from build123d import *

# Parameters (mm, degrees)
F1_DEPTH  = 3
F3_DEPTH  = 2
F4_R      = 1.5
F5_DEPTH  = 3
F6_SIZE   = 1
F7_R      = 1
F9_DEPTH  = 1.0010001
F10_R     = 1.49999
F11_W     = 6
F11_H     = 1.5
F12_DEPTH = 2.5


# Not quite as in the source:
# - a fillet or chamfer is up to 0.001 mm smaller than in the source, because OpenCascade refuses the exact size


with BuildPart() as f1:
    # F0 (on Top) → F1 (new body)
    with BuildSketch(Plane.XY):
        Polygon((4, 20), (-4, 20), (-4, 14.4568322948), (-17.7288018167, 0), (0, -18.8113879412), (17.1686839312, 0), (4, 14.4568322948), align=None)
    extrude(amount=F1_DEPTH)

    # F2 (on face) → F3 (cut)
    with BuildSketch(Plane.XY.offset(3)):
        with BuildLine():
            Line((1.5, 20), (-1.5, 20))
            Line((-1.5, 20), (-1.5, 10.3923048454))
            ThreePointArc((-1.5, 10.3923048454), (0, -10.5), (1.5, 10.3923048454))
            Line((1.5, 10.3923048454), (1.5, 20))
        make_face()
    extrude(amount=-F3_DEPTH, mode=Mode.SUBTRACT)

    # F4 (on face) → F5 (join)
    with BuildSketch(Plane.XY.offset(3)):
        with Locations((12.5, 0)):
            Circle(F4_R)
        with Locations((-12.5, 0)):
            Circle(F4_R)
        with Locations((0, -12.5)):
            Circle(F4_R)
    extrude(amount=F5_DEPTH)

    # F6
    f6_edges = [f1.edges().sort_by_distance(p)[0] for p in [
        (-14, 0, 6),
        (-1.5, -12.5, 6),
        (11, 0, 6),
    ]]
    chamfer(f6_edges, length=F6_SIZE)

    # F7
    f7_edges = [f1.edges().sort_by_distance(p)[0] for p in [
        (4, 17.228416, 0),
        (-4, 17.228416, 0),
        (-4, 14.456832, 1.5),
        (-10.864401, 7.228416, 0),
        (-4, 20, 1.5),
        (4, 14.456832, 1.5),
        (10.584342, 7.228416, 0),
        (4, 20, 1.5),
    ]]
    fillet(f7_edges, radius=F7_R)

    # F8 (on face) → F9 (cut, through all)
    with BuildSketch(Plane.XY.offset(1)):
        with BuildLine():
            Line((-1.5, 9.633924434), (-1.5, 9.8868599666))
            ThreePointArc((-1.5, 9.8868599666), (0, -10), (1.5, 9.8868599666))
            Line((1.5, 9.8868599666), (1.5, 9.633924434))
            ThreePointArc((1.5, 9.633924434), (0, -9.75), (-1.5, 9.633924434))
        make_face()
    extrude(amount=-F9_DEPTH, mode=Mode.SUBTRACT)

    # F10 (radius 1.5 in the source; OpenCascade refuses exactly that, so slightly less here)
    f10_edges = [f1.edges().sort_by_distance(p)[0] for p in [
        (1.5, 15.196152, 1),
        (-1.5, 15.196152, 1),
    ]]
    fillet(f10_edges, radius=F10_R)

    # F11 (on face) → F12 (cut)
    with BuildSketch(Plane.XY.offset(3)):
        with Locations((0, 14.75)):
            Rectangle(F11_W, F11_H)
    extrude(amount=-F12_DEPTH, mode=Mode.SUBTRACT)


solid = f1.part
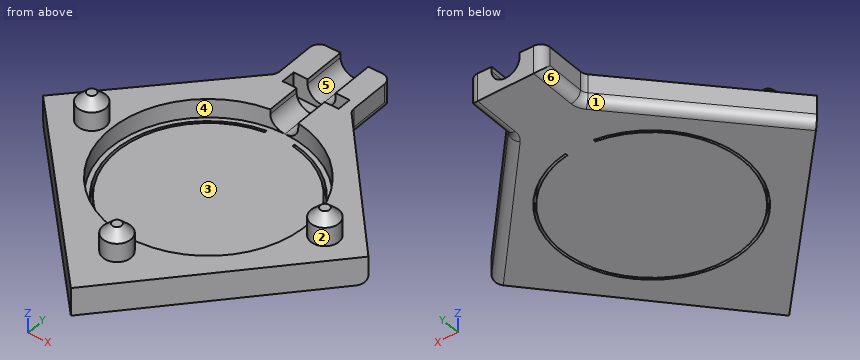
Read the model definition and answer for the solid it produces. Units are mm, in the model's axes. Face numbers are marked on the shaded views. A direction names the side the tool comes from. Coordinates: 2 decimals unless noted, no trailing zeros. Write each loop counter-clockwise with the first axis right and the second up, starting at its lowest first coordinate (ties: lowest second). Pieces come first, ordered by that corner, then holes. Notation, with made-up numbers: M 69,-30 L 93,-30 A24 cw 93,4 Z; hole C -13.75,50.25 d3. An arc over 180 degrees is marked long. Use a Markdown table: item, result.
Q1. The part is cut by section D-D, the plane x = 6. Give the number of separate pieces and of enclosed holes in the cut face, then the cut area to 3 significant figures.
Answer block:
| item | result |
|---|---|
| separate pieces | 3 |
| enclosed holes | 0 |
| area | 38.1 mm2 |
Q2. Determine the mould class of the marked faces 1, 2 and 3 for opening direction Y: released by +Y, released by -Y, zero draft, split by the parting line, or undercut.
Answer block:
| item | result |
|---|---|
| face 1 | released by +Y |
| face 2 | split by the parting line |
| face 3 | undercut |
Q3. The part is cut by section A-A, the plane y = -8.5. Write down the section's boundary in (x, z), then the cut area to 3 significant figures.
Answer block:
| item | result |
|---|---|
| outline | M -9.72,0 L -5.27,0 L -5.27,1 L -6.16,1 L -6.16,3 L -9.72,3 Z; M -4.78,0 L 4.78,0 L 4.78,1 L -4.78,1 Z; M 5.27,0 L 9.41,0 L 9.41,3 L 6.16,3 L 6.16,1 L 5.27,1 Z |
| area | 31.7 mm2 |
Q4. Each of these flat-tipped pins is pushed along its axis until it touches: pin 1 Ø10 at (x, y) = (-3.5, 14.5) entering from +Z; pin 2 Ø1.2 at (y, z) = (15, 1.5) entering from -X; pin 3 Ø0.6 at (y, z) = (16.5, 2.5) entering from -X. Where does it stop, or does it pass through?
Answer block:
| item | result |
|---|---|
| pin 1 | stops at z = 3 |
| pin 2 | stops at x = -4.11 |
| pin 3 | stops at x = -4 |
Q5. The part is cut by section C-C, the plane y = -12.5. Write down the section's boundary in (x, z).
Answer block:
| item | result |
|---|---|
| outline | M -5.95,0 L 5.76,0 L 5.76,3 L 1.5,3 L 1.5,5 L 0.5,6 L -0.5,6 L -1.5,5 L -1.5,3 L -5.95,3 Z |
Q6. Straight lines are drawn through the part: L1, parallel to Y at x = -1.5, z = 2; L2, parallel to Z at x = 11.5, y = 2.5; L3, parallel to Z at x = 1, y = 10. For each, find the intervals that lie inside material, in ascending order. Write a range as [from, to].
Answer block:
| item | result |
|---|---|
| L1 | y = [-17.22, -10.39], [10.39, 14], [15.5, 20] |
| L2 | z = [0, 3] |
| L3 | z = [0, 1] |
Q7. The part is cut by section B-B, the plane x = -2. Write down the section's boundary in (y, z), then the cut area to 3 significant figures.
Answer block:
| item | result |
|---|---|
| outline | M -16.69,0 L -9.8,0 L -9.8,1 L -10.31,1 L -10.31,3 L -16.69,3 Z; M -9.54,0 L 9.54,0 L 9.54,1 L -9.54,1 Z; M 9.8,0 L 20,0 L 20,3 L 15.5,3 L 15.5,0.5 L 14,0.5 L 14,3 L 10.31,3 L 10.31,1 L 9.8,1 Z |
| area | 64.6 mm2 |
Q8. Which of the six approach directions +Z, -Z, +X, -X, +Y, -Y give full straight-line access (tool end or side, diameter ignored) to the marked faces 4, 5 and 6?
Answer block:
| item | result |
|---|---|
| face 4 | +Z |
| face 5 | +Z, +Y |
| face 6 | -Z, -X, +Y |
